The listing builds one solid part. Answer for the finished solid, in the listing's coordinates (mm). A direction names the side the tool comes from. Round coordinates to 2 decimals unless told otherwise and drop trailing zeros. Write each loop counter-clockwise with the first axis right and the second up, starting at its lowest first coordinate (ties: lowest second). Pieces come first, ordered by that corner, then holes.
(1) The mould has two halves that part along X. Classify faces 1 (the face through (36, 4.514, 11)), 2 (the face through (-33.436, -1.81, -5.659)), 3 (the face through (-34.608, 0, 7)): +X half, -X half, draft (parallel to the pull), parting line (faces both ways), or undercut.
(2) Each of these flat-tipped pins is pushed along its axis until it touches: pin 1 Ø3 at (x, z) = (35, 12.5) entering from -Y; pin 2 Ø4.5 at (y, z) = (-11.5, -8.5) entering from +X; pin 3 Ø2 at (y, z) = (0.5, -5) entering from +X. Where does it stop, or does it pass through?
(3) A cutting plane is placed at A-A, the plane z = 13. Give the vertices of the cut face in (x, y).
(4) Find the intervals of material crossed by probe 1 along X at (y, z) = (-11.5, -8.5); probe 2 along X at (y, z) = (1.5, 9.5); probe 3 along Z at (x, y) = (-2, -2.5), in increasing order.
(5) For faces 4 (the face through (-18.28, -12.72, -8.38)), 5 (the face through (-18.28, -9.27, -9.99)), 6 (the face through (-33, 0, 14.986)), 7 (the face through (-34.563, -0.063, 18.117)), 8 (the face through (-17.026, -11, -9)), determine the directions among +Z, -Z, +X, -X, +Y, -Y from which every point of the face is accessible in a straight line to the end or side of a thin tool.
(6) A cutting plane is placed at C-C, the plane x = 28.5. Give the vertices of the cut face in (y, z) (3 decimals).
(7) A cutting plane is placed at D-D, the plane y = -13. Give the vertices of the cut face in (x, z), and give its area (3 significant figures).
(8) A cutting plane is placed at B-B, the plane x = 18.5. Give the vertices of the cut face in (y, z) (3 decimals).
from build123d import *

# Parameters (mm, degrees)
SKETCH1_W                      = 75.565
SKETCH1_H                      = 35.56
BOSS_EXTRUDE1_DEPTH            = 3.175
SKETCH6_W                      = 3.175
SKETCH6_H                      = 9.028368652
BOSS_EXTRUDE4_DEPTH            = 14.986
BOSS_EXTRUDE6_DEPTH            = 9.028368652
BOSS_EXTRUDE7_DEPTH            = 75.565
SKETCH10_W                     = 75.565
SKETCH10_H                     = 23.368
BOSS_EXTRUDE8_DEPTH            = 5.08
CUT_EXTRUDE1_DEPTH             = 82.008490267
CUT_EXTRUDE2_REACH             = 51.95
SKETCH12_W                     = 6.35
SKETCH12_H                     = 3.175
CUT_EXTRUDE2_DIRECTION_2_DEPTH = 50.950000932
CUT_EXTRUDE3_DEPTH             = 54.096105705
CUT_EXTRUDE4_REACH             = 55.451
SKETCH14_W                     = 2.54
SKETCH14_H                     = 3.81


with BuildPart() as part:
    # Sketch1 → Boss-Extrude1 (new body)
    with BuildSketch(Plane.XY):
        Rectangle(SKETCH1_W, SKETCH1_H)
    extrude(amount=-BOSS_EXTRUDE1_DEPTH)

    # Sketch6 → Boss-Extrude4 (add)
    with BuildSketch(Plane.XY):
        with Locations((-36.195, 0)):
            Rectangle(SKETCH6_W, SKETCH6_H)
        with Locations((36.195, 0)):
            Rectangle(SKETCH6_W, SKETCH6_H)
    extrude(amount=BOSS_EXTRUDE4_DEPTH)

    # Sketch8 → Boss-Extrude6 (add)
    with BuildSketch(Plane.XZ.offset(4.514184326)):
        Polygon((-37.7825, 14.986), (-31.4325, 14.986), (-37.7825, 21.336), align=None)
        Polygon((37.7825, 14.986), (31.4325, 14.986), (37.7825, 21.336), align=None)
    extrude(amount=-BOSS_EXTRUDE6_DEPTH)

    # Sketch9 → Boss-Extrude7 (add)
    with BuildSketch(Plane.ZY.offset(37.7825)):
        Polygon((-3.175, 17.78), (-16.795270199, 11.4287637), (-3.175, -17.78), align=None)
    extrude(amount=-BOSS_EXTRUDE7_DEPTH)

    # Sketch10 → Boss-Extrude8 (add)
    with BuildSketch(Plane(origin=(0, -4.391713703, -9.41806043), x_dir=(-1, 0, 0), z_dir=(0, -0.4226182617407007, -0.9063077870366493))):
        with Locations((0, -3.088339472)):
            Rectangle(SKETCH10_W, SKETCH10_H)
    extrude(amount=BOSS_EXTRUDE8_DEPTH)

    # Sketch11 → Cut-Extrude1 (cut, through all)
    with BuildSketch(Plane.ZY.offset(37.7825)):
        Polygon((-13.05074354, 3.398600367), (0, 4.514184326), (36.888684706, 18.275511072), (5.286071508, 25.150339228), (-30.3838484, 8.233222823), align=None)
        Polygon((-3.175, -17.78), (-7.689027521, -8.099636743), (0, -4.514184326), (40.158547499, -20.406390647), (15.599703883, -25.394905756), align=None)
    extrude(amount=-CUT_EXTRUDE1_DEPTH, mode=Mode.SUBTRACT)

    # Cut-Extrude2: up to this plane
    cut_extrude2_end = Plane(origin=(37.7825, -8.099636743, -7.689027521), z_dir=(0, 0.9063077870366495, -0.4226182617407008))
    # Sketch12 → Cut-Extrude2 (cut, up to the surface)
    with BuildSketch(Plane(origin=(0, 4.481438837, -0.38307559), x_dir=(1, 0, 0), z_dir=(0, 0.9963664433600627, -0.08516989225083536)), mode=Mode.PRIVATE) as cut_extrude2_sk1:
        with Locations((0, 4.378027407)):
            Rectangle(SKETCH12_W, SKETCH12_H)
    cut_extrude2_tool1 = split(extrude(cut_extrude2_sk1.sketch, amount=-CUT_EXTRUDE2_REACH, mode=Mode.PRIVATE), bisect_by=cut_extrude2_end, keep=Keep.BOTH, mode=Mode.PRIVATE)
    add(cut_extrude2_tool1.solids().sort_by_distance((0, 4.108563, -4.745195))[0], mode=Mode.SUBTRACT)

    # Sketch12 → Cut-Extrude2 direction 2 (cut)
    with BuildSketch(Plane(origin=(0, 4.481438837, -0.38307559), x_dir=(1, 0, 0), z_dir=(0, 0.9963664433600627, -0.08516989225083536))):
        with Locations((0, 4.378027407)):
            Rectangle(SKETCH12_W, SKETCH12_H)
    extrude(amount=CUT_EXTRUDE2_DIRECTION_2_DEPTH, mode=Mode.SUBTRACT)

    # Sketch13 → Cut-Extrude3 (cut, through all)
    with BuildSketch(Plane(origin=(0, 7.790314071, -3.632683111), x_dir=(1, 0, 0), z_dir=(0, 0.9063077870366493, -0.4226182617407007))):
        Polygon((-29.21, 10.391679918), (-37.7825, 1.267223267), (-37.7825, 11.639630657), (-37.7825, 15.471679918), (-29.21, 15.471679918), align=None)
        Polygon((37.7825, 1.267223267), (37.7825, 11.639630657), (37.7825, 15.471679918), (29.21, 15.471679918), (29.21, 10.391679918), align=None)
    extrude(amount=-CUT_EXTRUDE3_DEPTH, mode=Mode.SUBTRACT)

    # Sketch14 → Cut-Extrude4 (cut, up to next)
    with BuildSketch(Plane(origin=(0, -6.538614473, -14.022103988), x_dir=(-1, 0, 0), z_dir=(0, -0.4226182617407007, -0.9063077870366494)), mode=Mode.PRIVATE) as cut_extrude4_sk1:
        with Locations((-18.050542255, -6.082892111)):
            Rectangle(SKETCH14_W, SKETCH14_H)
    cut_extrude4_tool1 = extrude(cut_extrude4_sk1.sketch, amount=-CUT_EXTRUDE4_REACH, mode=Mode.PRIVATE) & part.part
    # Sketch14 → Cut-Extrude4 (cut, up to next)
    with BuildSketch(Plane(origin=(0, -6.538614473, -14.022103988), x_dir=(-1, 0, 0), z_dir=(0, -0.4226182617407007, -0.9063077870366494)), mode=Mode.PRIVATE) as cut_extrude4_sk2:
        with Locations((18.295855998, -6.082892111)):
            Rectangle(SKETCH14_W, SKETCH14_H)
    cut_extrude4_tool2 = extrude(cut_extrude4_sk2.sketch, amount=-CUT_EXTRUDE4_REACH, mode=Mode.PRIVATE) & part.part
    add(cut_extrude4_tool1.solids().sort_by_distance((18.050542, -12.051587, -11.451363))[0], mode=Mode.SUBTRACT)
    add(cut_extrude4_tool2.solids().sort_by_distance((-18.295856, -12.051587, -11.451363))[0], mode=Mode.SUBTRACT)


solid = part.part
Solutions:
1. face 1: draft
1. face 2: -X half
1. face 3: undercut
2. pin 1: stops at y = -4.51
2. pin 2: stops at x = 29.21
2. pin 3: stops at x = 35.85
3. outline: (-37.78, -4.51) - (-34.61, -4.51) - (-34.61, 4.51) - (-37.78, 4.51) - close; (34.61, -4.51) - (37.78, -4.51) - (37.78, 4.51) - (34.61, 4.51) - close
4. probe 1: x = -29.21 to -19.57, -17.03 to 16.78, 19.32 to 29.21
4. probe 2: x = -37.78 to -34.61, 34.61 to 37.78
4. probe 3: z = -15.91 to -5.77, -2.59 to 0
5. face 4: -Z
5. face 5: +Z
5. face 6: +Y, -Y
5. face 7: +Z, +Y, -Y
5. face 8: none
6. outline: (-19.927, -7.779) - (1.252, -17.655) - (3.399, -13.051) - (4.514, 0) - (-4.514, 0) - (-8.1, -7.689) - (-17.78, -3.175) - close
7. outline: (-29.21, -11.01) - (-19.57, -11.01) - (-19.57, -8.98) - (-17.03, -8.98) - (-17.03, -11.01) - (16.78, -11.01) - (16.78, -8.98) - (19.32, -8.98) - (19.32, -11.01) - (29.21, -11.01) - (29.21, -5.4) - (-29.21, -5.4) - close
7. area: 317 mm2
8. outline: (-19.927, -7.779) - (-13.778, -10.646) - (-11.631, -6.042) - (-17.78, -3.175) - close; (-10.325, -12.256) - (1.252, -17.655) - (3.399, -13.051) - (4.514, 0) - (-4.514, 0) - (-8.1, -7.689) - (-8.178, -7.652) - close
